```python
from build123d import *

# Parameters (mm, degrees)
SKETCH1_W           = 83
SKETCH1_H           = 58
BOSS_EXTRUDE1_DEPTH = 21.92
SHELL1_T            = -2
SKETCH2_R           = 2
BOSS_EXTRUDE2_DEPTH = 6
SKETCH3_W           = 12.74
SKETCH3_H           = 4.96
SKETCH3_W_2         = 13
SKETCH3_H_2         = 13
CUT_EXTRUDE1_DEPTH  = 2


with BuildPart() as part:
    # Sketch1 → Boss-Extrude1 (new body)
    with BuildSketch(Plane(origin=(0, 0, 0), x_dir=(0, 1, 0), z_dir=(0, 0, 1))):
        Rectangle(SKETCH1_W, SKETCH1_H)
    extrude(amount=BOSS_EXTRUDE1_DEPTH)

    # Shell1
    shell1_openings = [part.faces().sort_by_distance(p)[0] for p in [
        (0, 0, 21.92),
    ]]
    offset(amount=SHELL1_T, openings=shell1_openings, kind=Kind.INTERSECTION)

    # Sketch2 → Boss-Extrude2 (add)
    # profile 1 of 4: a face of its own
    with BuildSketch(Plane.XY.offset(2)):
        with BuildLine():
            Line((-27, 39.5), (-18, 39.5))
            Line((-18, 39.5), (-18, 34.5))
            ThreePointArc((-18, 34.5), (-19.171572875, 31.671572875), (-22, 30.5))
            Line((-22, 30.5), (-27, 30.5))
            Line((-27, 30.5), (-27, 39.5))
        make_face()
        with Locations((-22, 34.5)):
            Circle(SKETCH2_R, mode=Mode.SUBTRACT)
    # profile 2 of 4: a face of its own
    with BuildSketch(Plane.XY.offset(2)):
        with BuildLine():
            Line((18, 39.5), (18, 34.5))
            ThreePointArc((18, 34.5), (19.171572875, 31.671572875), (22, 30.5))
            Line((22, 30.5), (27, 30.5))
            Line((27, 30.5), (27, 39.5))
            Line((27, 39.5), (18, 39.5))
        make_face()
        with Locations(Location((22, 34.5, 0), (0, 0, 180))):
            Circle(SKETCH2_R, mode=Mode.SUBTRACT)
    # profile 3 of 4: a face of its own
    with BuildSketch(Plane.XY.offset(2)):
        with BuildLine():
            Line((27, -39.5), (18, -39.5))
            Line((18, -39.5), (18, -34.5))
            ThreePointArc((18, -34.5), (19.171572875, -31.671572875), (22, -30.5))
            Line((22, -30.5), (27, -30.5))
            Line((27, -30.5), (27, -39.5))
        make_face()
        with Locations((22, -34.5)):
            Circle(SKETCH2_R, mode=Mode.SUBTRACT)
    # profile 4 of 4: a face of its own
    with BuildSketch(Plane.XY.offset(2)):
        with BuildLine():
            Line((-18, -39.5), (-18, -34.5))
            ThreePointArc((-18, -34.5), (-19.171572875, -31.671572875), (-22, -30.5))
            Line((-22, -30.5), (-27, -30.5))
            Line((-27, -30.5), (-27, -39.5))
            Line((-27, -39.5), (-18, -39.5))
        make_face()
        with Locations(Location((-22, -34.5, 0), (0, 0, 180))):
            Circle(SKETCH2_R, mode=Mode.SUBTRACT)
    extrude(amount=BOSS_EXTRUDE2_DEPTH)

    # Sketch3 → Cut-Extrude1 (cut)
    with BuildSketch(Plane.XZ.offset(41.5)):
        with Locations((-12.08, 11.93)):
            Rectangle(SKETCH3_W, SKETCH3_H)
        with Locations((12, 15.95)):
            Rectangle(SKETCH3_W_2, SKETCH3_H_2)
    extrude(amount=-CUT_EXTRUDE1_DEPTH, mode=Mode.SUBTRACT)


solid = part.part
```
Model file for the job. Use its own axes, mm. A direction names the side the tool comes from. Give positions to 0.01 mm unless a question says otherwise; leave off trailing zeros. Write each loop counter-clockwise with the first axis right and the second up, starting at its lowest first coordinate (ties: lowest second). Pieces come first, ordered by that corner, then holes. Notation, with made-up numbers: M -11,-19 L -7,-19 A30 ccw -7,10 Z; hole C 61.25,8.5 d10. An arc over 180 degrees is marked long. Use a Markdown table: item, result.
1) Cut at B-B (z = 4). List the corners of the cut face in (x, y), and give its area (3 significant figures).
Responses:
| item | result |
|---|---|
| outline | M -29,-41.5 L 29,-41.5 L 29,41.5 L -29,41.5 Z; hole M -27,-30.5 L -22,-30.5 A4 cw -18,-34.5 L -18,-39.5 L 18,-39.5 L 18,-34.5 A4 cw 22,-30.5 L 27,-30.5 L 27,30.5 L 22,30.5 A4 cw 18,34.5 L 18,39.5 L -18,39.5 L -18,34.5 A4 cw -22,30.5 L -27,30.5 Z; hole C -22,-34.5 d4; hole C -22,34.5 d4; hole C 22,-34.5 d4; hole C 22,34.5 d4 |
| area | 808 mm2 |
2) Cut at A-A (x = 7). List the corners of the cut face in (y, z).
Responses:
| item | result |
|---|---|
| outline | M -41.5,0 L 41.5,0 L 41.5,21.92 L 39.5,21.92 L 39.5,2 L -39.5,2 L -39.5,9.45 L -41.5,9.45 Z |
3) Drill centre lines: line 1 (Y direction, x = -22, z = 4.9); line 2 (X direction, y = 34, z = 20); line 3 (Y direction, x = -10.5, z = 9). Where is each one in solid material? Low to high. Write a range as from..to.
Responses:
| item | result |
|---|---|
| line 1 | y = -41.5..-36.5, -32.5..-30.5, 30.5..32.5, 36.5..41.5 |
| line 2 | x = -29..-27, 27..29 |
| line 3 | y = -41.5..-39.5, 39.5..41.5 |
4) Pull direction X, two halves, no side cores. Call faces 6 (the flat face through (-12, -41, 14.41)), 7 (the flat face through (-22, 34, 2)), 8 (the flat face through (0, 41.5, 11)): +X half, -X half, draft (parallel to the pull), parting line (faces both ways), or undercut.
Responses:
| item | result |
|---|---|
| face 6 | undercut |
| face 7 | undercut |
| face 8 | draft |
5) Cut at C-C (x = -15). List the corners of the cut face in (y, z).
Responses:
| item | result |
|---|---|
| outline | M -41.5,0 L 41.5,0 L 41.5,21.92 L 39.5,21.92 L 39.5,2 L -39.5,2 L -39.5,9.45 L -41.5,9.45 Z; M -41.5,14.41 L -39.5,14.41 L -39.5,21.92 L -41.5,21.92 Z |
6) Tool access for faces 1 (the flat face through (-5.71, -41, 12)), 2 (the flat face through (0, -41.5, 11)), 3 (the flat face through (0, -1, 2)), 4 (the flat face through (18.5, -41, 16)), 5 (the flat face through (28, 3, 21.92)): list every direction of +Z, -Z, +X, -X, +Y, -Y with a clear straight run to the whole face (end or side of a thin tool).
Responses:
| item | result |
|---|---|
| face 1 | -Y |
| face 2 | +Z, -Z, +X, -X, -Y |
| face 3 | +Z |
| face 4 | +Z, -Y |
| face 5 | +Z, +X, -X, +Y, -Y |
7) Pin check, flat tips, straight feed: pin 1 (3.5 mm diameter, centred on x = -22, y = 34.5, fed in from -Z); pin 2 (2.5 mm diameter, centred on x = -24, y = 34.5, fed in from +Z); pin 3 (2 mm diameter, centred on x = 11, y = -40.5, fed in from +Z); pin 4 (5 mm diameter, centred on x = -1.5, y = 3, fed in from +Z). Stop position of each tip, or through.
Responses:
| item | result |
|---|---|
| pin 1 | stops at z = 0 |
| pin 2 | stops at z = 8 |
| pin 3 | stops at z = 9.45 |
| pin 4 | stops at z = 2 |
8) Cut at D-D (y = 12.5). List the corners of the cut face in (x, z).
Responses:
| item | result |
|---|---|
| outline | M -29,0 L 29,0 L 29,21.92 L 27,21.92 L 27,2 L -27,2 L -27,21.92 L -29,21.92 Z |
